Autodesk Inventor part; units mm, degrees
ref_plane "YZ Plane" through (0, 0, 0) normal (1, 0, 0) x (0, 1, 0)
ref_plane "XZ Plane" through (0, 0, 0) normal (0, 1, 0) x (-1, 0, 0)
ref_plane "XY Plane" through (0, 0, 0) normal (0, 0, 1) x (1, 0, 0)
sketch "Sketch_5" plane through (0, 0, 0) normal (0, 0, 1) x (1, 0, 0)
  line L0 (-10, 9) -> (-10, 3.3)
  arc A0 (-10, 3.3) -> (-9.7, 3) centre (-9.7, 3.3) ccw
  line L1 (-9.7, 3) -> (-8, 3)
  line L2 (-8, 3) -> (-8, 6)
  line L3 (-8, 6) -> (-7.0607, 6)
  line L4 (-7.0607, 6) -> (-4, 2.9393)
  line L5 (-4, 2.9393) -> (-4, 0.3)
  line L6 (-4, 0.3) -> (-3.7, 0)
  line L7 (-3.7, 0) -> (-4, -0.3)
  line L8 (-4, -0.3) -> (-4, -2.9393)
  line L9 (-4, -2.9393) -> (-7.0607, -6)
  line L10 (-7.0607, -6) -> (-8, -6)
  line L11 (-8, -6) -> (-8, -3)
  line L12 (-8, -3) -> (-9.7, -3)
  arc A1 (-9.7, -3) -> (-10, -3.3) centre (-9.7, -3.3) ccw
  line L13 (-10, -3.3) -> (-10, -9)
  arc A2 (-10, -9) -> (-9, -10) centre (-9, -9) ccw
  line L14 (-9, -10) -> (-3.3, -10)
  arc A3 (-3.3, -10) -> (-3, -9.7) centre (-3.3, -9.7) ccw
  line L15 (-3, -9.7) -> (-3, -8)
  line L16 (-3, -8) -> (-6, -8)
  line L17 (-6, -8) -> (-6, -7.0607)
  line L18 (-6, -7.0607) -> (-2.9393, -4)
  line L19 (-2.9393, -4) -> (-0.3, -4)
  line L20 (-0.3, -4) -> (0, -3.7)
  line L21 (0, -3.7) -> (0.3, -4)
  line L22 (0.3, -4) -> (2.9393, -4)
  line L23 (2.9393, -4) -> (6, -7.0607)
  line L24 (6, -7.0607) -> (6, -8)
  line L25 (6, -8) -> (3, -8)
  line L26 (3, -8) -> (3, -9.7)
  arc A4 (3, -9.7) -> (3.3, -10) centre (3.3, -9.7) ccw
  line L27 (3.3, -10) -> (9, -10)
  arc A5 (9, -10) -> (10, -9) centre (9, -9) ccw
  line L28 (10, -9) -> (10, -3.3)
  arc A6 (10, -3.3) -> (9.7, -3) centre (9.7, -3.3) ccw
  line L29 (9.7, -3) -> (8, -3)
  line L30 (8, -3) -> (8, -6)
  line L31 (8, -6) -> (7.0607, -6)
  line L32 (7.0607, -6) -> (4, -2.9393)
  line L33 (4, -2.9393) -> (4, -0.3)
  line L34 (4, -0.3) -> (3.7, 0)
  line L35 (3.7, 0) -> (4, 0.3)
  line L36 (4, 0.3) -> (4, 2.9393)
  line L37 (4, 2.9393) -> (7.0607, 6)
  line L38 (7.0607, 6) -> (8, 6)
  line L39 (8, 6) -> (8, 3)
  line L40 (8, 3) -> (9.7, 3)
  arc A7 (9.7, 3) -> (10, 3.3) centre (9.7, 3.3) ccw
  line L41 (10, 3.3) -> (10, 9)
  arc A8 (10, 9) -> (9, 10) centre (9, 9) ccw
  line L42 (9, 10) -> (3.3, 10)
  arc A9 (3.3, 10) -> (3, 9.7) centre (3.3, 9.7) ccw
  line L43 (3, 9.7) -> (3, 8)
  line L44 (3, 8) -> (6, 8)
  line L45 (6, 8) -> (6, 7.0607)
  line L46 (6, 7.0607) -> (2.9393, 4)
  line L47 (2.9393, 4) -> (0.3, 4)
  line L48 (0.3, 4) -> (0, 3.7)
  line L49 (0, 3.7) -> (-0.3, 4)
  line L50 (-0.3, 4) -> (-2.9393, 4)
  line L51 (-2.9393, 4) -> (-6, 7.0607)
  line L52 (-6, 7.0607) -> (-6, 8)
  line L53 (-6, 8) -> (-3, 8)
  line L54 (-3, 8) -> (-3, 9.7)
  arc A10 (-3, 9.7) -> (-3.3, 10) centre (-3.3, 9.7) ccw
  line L55 (-3.3, 10) -> (-9, 10)
  arc A11 (-9, 10) -> (-10, 9) centre (-9, 9) ccw
  circle A12 centre (0, 0) radius 2.1
extrude "Extrusion1" add sketch "Sketch_5" against normal blind 220
properties part number "KHFS5-2020-4000" material "Aluminum 6061"
For this review, take the finished solid that the model builds, in its own axes (mm). Round coordinates to 2 decimals unless told otherwise and drop trailing zeros. Write item = value, one per line. Start each with the question number.
1) The part is to be moulded in two halves that separate along X. For faces 1 (the face through (-10, -6, -108)), 2 (the face through (2.003, 0.631, -108.46)), 3 (the face through (10, -6, -108)), 4 (the face through (6, 10, -108)), say which applies: +X half, -X half, draft (parallel to the pull), parting line (faces both ways), or undercut.
2) Insertion check: pin 1 (3 mm diameter, centred on y = 0.5, z = -55, fed in from +X); pin 2 (1.3 mm diameter, centred on y = 1.5, z = -104, fed in from -X); pin 3 (1.5 mm diameter, centred on x = -2.5, z = -67, fed in from +Y). Each pin has a flat end and moves straight along its axis. Give the tip position at first contact, or say it passes through.
3) To check wall thickness, follow line 1 (Y direction, x = 0, z = -62.5); line 2 (X direction, y = 7.5, z = -93); line 3 (Y direction, x = 4.5, z = -117). State the ranges of each line that lie inside material, in increasing order. Write a range as from..to.
Verdict:
q1.face_1 = -X half
q1.face_2 = undercut
q1.face_3 = +X half
q1.face_4 = draft
q2.pin_1 = 4
q2.pin_2 = -4
q2.pin_3 = 10
q3.line_1 = -3.7..-2.1, 2.1..3.7
q3.line_2 = -10..-6, 6..10
q3.line_3 = -10..-8, -5.56..-3.44, 3.44..5.56, 8..10
